Geometry: final body of the model. Coordinates: model frame, mm. A direction names the side the tool comes from. Give positions to 0.01 mm unless a question says otherwise; leave off trailing zeros. Order: outer loops, then holes, each group sorted by start corner. A loop starts at its lowest first (then second) coordinate and runs counter-clockwise, first axis right, second up. Notation, with made-up numbers: (75.25, -0.5) - (133.25, -0.5) arc R22 ccw to (133.25, 21.5) - close; hole circle Ø2 at (10, 44). An arc over 180 degrees is marked (long way). Use one line per item in the form item = value.
from build123d import *

# Parameters (mm, degrees)
F0_R     = 11
F1_DEPTH = 2
F2_R     = 3.9
F3_DEPTH = 6
F4_R     = 0.5


# Not quite as in the source:
# - a feature names something its author has since deleted; it is built from what else it names


with BuildPart() as f1:
    # F0 (on Top) → F1 (new body)
    with BuildSketch(Plane.XY):
        Circle(F0_R)
    extrude(amount=F1_DEPTH)

    # F2 (on Top) → F3 (join)
    with BuildSketch(Plane.XY):
        Circle(F2_R)
    extrude(amount=F3_DEPTH)

    # F4
    f4_edges = [f1.edges().sort_by_distance(p)[0] for p in [
        (-11, 0, 2),
        (-11, 0, 0),
        (-3.9, 0, 6),
    ]]
    fillet(f4_edges, radius=F4_R)


solid = f1.part
(1) Contact query for flat-ended pins moving along their axis: pin 1 Ø4 at (x, y) = (-4.5, -4.5) entering from +Z; pin 2 Ø3 at (x, z) = (5, 1.5) entering from -Y. Output: stop coordinate, or through.
Computed values:
pin_1 = 2
pin_2 = -10.43
(2) Cut plane C-C on z = 1.15. Output: boundary loops of the cut face in (x, y), plus the area to 3 significant figures.
Computed values:
outline = circle Ø22 at (0, 0)
area = 380 mm²
(3) Ray query, line 1 along Z through (x, y) = (6.25, -0.5); line 2 along X through (y, z) = (-1, 1.35); line 3 along X through (y, z) = (6.25, 0.55). Return the intervals inside material, ascending.
Computed values:
line_1 = 0 to 2
line_2 = -10.95 to 10.95
line_3 = -9.05 to 9.05
(4) Reachability of faces 1 (the face through (5, 0, 2)), 2 (the face through (0, 0, 6)) from +Z, -Z, +X, -X, +Y, -Y: full face, straight path, thin tool, end or side. Return the list, or none.
Computed values:
face_1 = +Z
face_2 = +Z, +X, -X, +Y, -Y
(5) Cut plane A-A on x = 0. Output: boundary loops of the cut face in (y, z), plus the area to 3 significant figures.
Computed values:
outline = (-11, 0.5) arc R0.5 ccw to (-10.5, 0) - (10.5, 0) arc R0.5 ccw to (11, 0.5) - (11, 1.5) arc R0.5 ccw to (10.5, 2) - (3.9, 2) - (3.9, 5.5) arc R0.5 ccw to (3.4, 6) - (-3.4, 6) arc R0.5 ccw to (-3.9, 5.5) - (-3.9, 2) - (-10.5, 2) arc R0.5 ccw to (-11, 1.5) - close
area = 74.9 mm²
